The listing builds one solid part. Answer for the finished solid, in the listing's coordinates (mm). A direction names the side the tool comes from. Coordinates: 2 decimals unless noted, no trailing zeros. Loops run counter-clockwise (first coordinate to the right, second up) from the corner with the lowest first, then second, coordinate; pieces in that order, holes last. Notation, with made-up numbers: (60.25, 7) - (117.25, 7) arc R38 cw to (117.25, 46) - close; hole circle Ø7 at (-36.5, -25). An arc over 180 degrees is marked (long way). Write each question's results on one line, items separated by ' | '. Start each with the question number.
(1) Find section B-B on x = -12.5. Determine the outline of the cut face in (y, z), then the cut area to 3 significant figures.
(2) Consider line 1 (X direction, y = 11.5, z = 3); line 2 (X direction, y = 18, z = -6); line 3 (Y direction, x = 25, z = 3.5). Determine where each line is inside the solid, lowest interval first. Write a range as from..to.
(3) Determine the mould class of faces 1 (the cylindrical face through (25.3, 18.8, 1.8)), 2 (the cylindrical face through (0.05, 10.14, -22.67)), 3 (the flat face through (22.287, 19, 3)), 4 (the flat face through (27, 19, 0)) for opening direction Z: released by +Z, released by -Z, zero draft, split by the parting line, or undercut.
(4) For faces 5 (the flat face through (32.287, 10, -3)), 6 (the flat face through (0, 10, -20.171)), 7 (the flat face through (-15, 10, -20.171)), 8 (the flat face through (-22.287, 19, 3)), determine the directions among +Z, -Z, +X, -X, +Y, -Y from which every point of the face is accessible in a straight line to the end or side of a thin tool.
(5) Find section A-A on x = 0. Determine the outline of the cut face in (y, z), then the cut area to 3 significant figures.
(6) Find section D-D on z = -18.5. Determine the outline of the cut face in (x, y), then the cut area to 3 significant figures.
(7) Given pin 1 Ø5 at (y, z) = (4.5, -5.5) entering from +X; pin 2 Ø5 at (x, y) = (26.5, 11.5) entering from -Z; pin 3 Ø12 at (y, z) = (9, -5.5) entering from -X, each flat-ended and moving along its own axis, determine where each tip first touches the part or whether it passes through.
(8) Find section C-C on y = 1.5. State how many separate pieces and enclosed holes the cut face has, then the cut area to 3 significant figures.
from build123d import *

# Parameters (mm, degrees)
EXTRUDE_1_DEPTH     = 20
SKETCH_2_W          = 10
SKETCH_2_H          = 8
SKETCH_2_R          = 1.5
EXTRUDE_2_DEPTH     = 20
SKETCH_3_W          = 10
SKETCH_3_H          = 15
CUT_EXTRUDE_1_DEPTH = 6.5
CHAMFER_1_SIZE      = 3
FILLET_1_R          = 2
FILLET_2_R          = 1.5
EXTRUDE_3_DEPTH     = 20


with BuildPart() as part:
    # 草图1 → 凸台-拉伸1 (new body)
    with BuildSketch(Plane(origin=(0, 0, 0), x_dir=(1, 0, 0), z_dir=(0, 1, 0))):
        with BuildLine():
            Line((-52.384848004, 0), (-49.769696007, 0))
            ThreePointArc((-49.769696007, 0), (-45, -6.5), (-40.230303993, 0))
            Line((-40.230303993, 0), (-35.115151996, 0))
            Line((-35.115151996, 0), (-35.115151996, 11.078445968))
            Line((-35.115151996, 11.078445968), (-27.310228331, 20.17100506))
            Line((-27.310228331, 20.17100506), (27.310228331, 20.17100506))
            Line((27.310228331, 20.17100506), (35.115151996, 11.078445968))
            Line((35.115151996, 11.078445968), (35.115151996, 0))
            Line((35.115151996, 0), (40.230303993, 0))
            ThreePointArc((40.230303993, 0), (45, -6.5), (49.769696007, 0))
            Line((49.769696007, 0), (52.384848004, 0))
            Line((52.384848004, 0), (55, 0))
            Line((55, 0), (55, -8))
            Line((55, -8), (32.287206254, -8))
            Line((32.287206254, -8), (32.287206254, 10.811768263))
            Line((32.287206254, 10.811768263), (26.82852765, 17.17100506))
            Line((26.82852765, 17.17100506), (-26.82852765, 17.17100506))
            Line((-26.82852765, 17.17100506), (-32.287206254, 10.811768263))
            Line((-32.287206254, 10.811768263), (-32.287206254, -8))
            Line((-32.287206254, -8), (-55, -8))
            Line((-55, -8), (-55, 0))
            Line((-55, 0), (-52.384848004, 0))
        make_face()
    extrude(amount=EXTRUDE_1_DEPTH)

    # 草图2 → 凸台-拉伸2 (add)
    with BuildSketch(Plane(origin=(0, 20, 0), x_dir=(1, 0, 0), z_dir=(0, 1, 0))):
        with Locations((-27.287206254, -4)):
            Rectangle(SKETCH_2_W, SKETCH_2_H)
        with Locations(Location((-26.787206254, -2, 0), (0, 0, 270))):
            Circle(SKETCH_2_R, mode=Mode.SUBTRACT)
    extrude(amount=-EXTRUDE_2_DEPTH)

    # 草图3 → 切除-拉伸1 (cut)
    with BuildSketch(Plane(origin=(0, 0, 0), x_dir=(-1, 0, 0), z_dir=(0, 0, -1))):
        with Locations((27.287206254, 10.122040723)):
            Rectangle(SKETCH_3_W, SKETCH_3_H)
    extrude(amount=-CUT_EXTRUDE_1_DEPTH, mode=Mode.SUBTRACT)

    # 镜向1: part across plane


with BuildPart() as part_1:
    add(part.part)
    add(part.part.mirror(Plane.ZY))

    # 倒角1
    # the kernel refuses this chamfer: 3 mm, written as the material it takes off along each edge
    with BuildSketch(Plane(origin=(22.287206254, 27.715048964, 8), x_dir=(-0.027495876610587933, 0, -0.9996219169112968), z_dir=(0, -1, 0)), Plane(origin=(-22.287206254, 27.715048964, 8), x_dir=(-0.9996219169112968, 0, 0.02749587661058619), z_dir=(0, -1, 0))) as chamfer_1_piece_1:
        Polygon((CHAMFER_1_SIZE * 0.999621916911, CHAMFER_1_SIZE * 0.0274958766106), (-CHAMFER_1_SIZE * 0.0274958766106, CHAMFER_1_SIZE * 0.999621916911), (0, 0), align=None)
    extrude(amount=35.430097928, mode=Mode.SUBTRACT)
    with BuildSketch(Plane(origin=(55, -7.715048964, 8), x_dir=(-0.9996219169112965, 0, 0.02749587661058705), z_dir=(0, 1, 0)), Plane(origin=(-55, -7.715048964, 8), x_dir=(-0.027495876610586775, 0, -0.9996219169112968), z_dir=(0, 1, 0))) as chamfer_1_piece_2:
        Polygon((CHAMFER_1_SIZE * 0.999621916911, -CHAMFER_1_SIZE * 0.0274958766106), (-CHAMFER_1_SIZE * 0.0274958766106, -CHAMFER_1_SIZE * 0.999621916911), (0, 0), align=None)
    extrude(amount=35.430097928, mode=Mode.SUBTRACT)

    # 圆角1
    fillet_1_edges = [part_1.edges().sort_by_distance(p)[0] for p in [
        (32.287206254, 10.122040723, 6.5),
        (55, 10, 0),
        (-55, 10, 0),
        (-35.115151996, 10, 0),
        (35.115151996, 10, 0),
        (-32.287206254, 10.122040723, 6.5),
    ]]
    fillet(fillet_1_edges, radius=FILLET_1_R)

    # 圆角2
    fillet_2_edges = [part_1.edges().sort_by_distance(p)[0] for p in [
        (22.287206254, 1.311020362, 0),
        (32.287206254, 1.311020362, 0),
        (32.287206254, 18.811020362, 0),
        (22.287206254, 18.811020362, 0),
        (-22.287206254, 1.311020362, 0),
        (-32.287206254, 1.311020362, 0),
        (-32.287206254, 18.811020362, 0),
        (-22.287206254, 18.811020362, 0),
    ]]
    fillet(fillet_2_edges, radius=FILLET_2_R)

    # 草图4 → 凸台-拉伸3 (add)
    with BuildSketch(Plane(origin=(0, 20, 0), x_dir=(1, 0, 0), z_dir=(0, 1, 0))):
        with BuildLine():
            Line((-2.5, 20.17100506), (-1.25, 20.17100506))
            ThreePointArc((-1.25, 20.17100506), (0, 21.42100506), (1.25, 20.17100506))
            Line((1.25, 20.17100506), (2.5, 20.17100506))
            ThreePointArc((2.5, 20.17100506), (0, 22.67100506), (-2.5, 20.17100506))
        make_face()
    extrude(amount=-EXTRUDE_3_DEPTH)


solid = part_1.part
Values:
1) outline: (0, -20.17) - (20, -20.17) - (20, -17.17) - (0, -17.17) - close | area: 60.0 mm²
2) line 1: x = -55..-49.77, -40.23..-32.29, 32.29..40.23, 49.77..55 | line 2: x = -35.12..-32.29, 32.29..35.12 | line 3: y = 0..2.62, 17.62..20
3) face 1: undercut | face 2: released by -Z | face 3: zero draft | face 4: undercut
4) face 5: none | face 6: +Y, -Y | face 7: -Z, -X, +Y, -Y | face 8: +Z, +Y, -Y
5) outline: (0, -22.67) - (20, -22.67) - (20, -21.42) - (0, -21.42) - close; (0, -20.17) - (20, -20.17) - (20, -17.17) - (0, -17.17) - close | area: 85.0 mm²
6) outline: (-28.74, 0) - (28.74, 0) - (28.74, 20) - (-28.74, 20) - close | area: 1,150 mm²
7) pin 1: stops at x = 35.12 | pin 2: stops at z = -20.17 | pin 3: stops at x = -54.32
8) separate pieces: 1 | enclosed holes: 3 | area: 662 mm²
